Check sheet for the modelled part. Datum: model origin and axes. Units: mm. Face numbers are marked on the shaded views. A direction names the side the tool comes from. Give positions to 0.01 mm unless a question says otherwise; leave off trailing zeros. Order: outer loops, then holes, each group sorted by start corner. A loop starts at its lowest first (then second) coordinate and runs counter-clockwise, first axis right, second up.
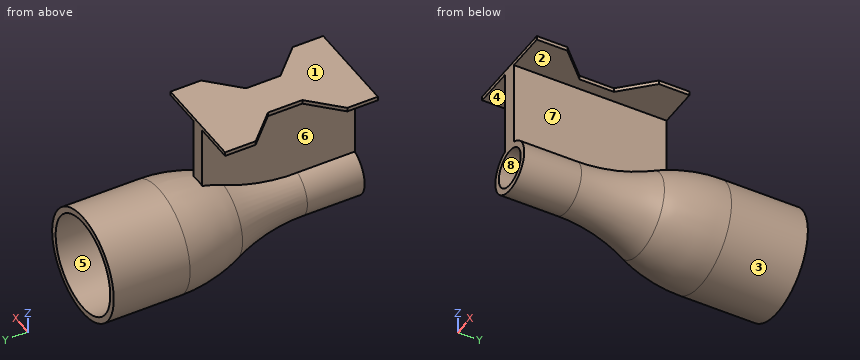
Autodesk Inventor part; units mm, degrees
ref_plane "YZ Plane" through (0, 0, 0) normal (1, 0, 0) x (0, 1, 0)
ref_plane "XZ Plane" through (0, 0, 0) normal (0, 1, 0) x (-1, 0, 0)
ref_plane "XY Plane" through (0, 0, 0) normal (0, 0, 1) x (1, 0, 0)
sketch "Szkic1" plane through (0, 0, 0) normal (1, 0, 0) x (0, 1, 0)
  line L0 (70, 12.5) -> (50, 12.5)
  arc A0 (50, 12.5) -> (35, 9.2857) centre (50, -24.1071) ccw
  arc A1 (15, 5) -> (35, 9.2857) centre (15, 53.8095) ccw
  line L1 (15, 5) -> (0, 5)
  line L2 (0.9785, 0) -> (128.1793, 0) construction
  line L3 (70, 14.1) -> (50, 14.1)
  arc A2 (50, 14.1) -> (34.3444, 10.7452) centre (50, -24.1071) ccw
  arc A3 (15, 6.6) -> (34.3444, 10.7452) centre (15, 53.8095) ccw
  line L4 (15, 6.6) -> (0, 6.6)
  line L5 (70, 14.1) -> (70, 12.5)
  line L6 (0, 6.6) -> (0, 5)
  line L7 (-25.6359, 0) -> (153.8152, 0)
  line L8 (70, 14.1) -> (70, 0)
  line L9 (0, 0) -> (0, 5)
  dimension "d35" = 5
  dimension "d36" = 12.5
  dimension "d37" = 70
  dimension "d38" = 20
  dimension "d39" = 15
  dimension "d40" = 20
  dimension "d41" = 1.6
revolve "Obrót1" add sketch "Szkic1" angle 360 about axis through (0, -10, 0) along (0, 1, 0) contours L0 A0 A1 L1 L6 L4 A3 A2 L3 L5
sketch "Szkic3" plane through (0, 0, 0) normal (0, 1, 0) x (-1, 0, 0)
  line L0 (2.1408, 6.3327) -> (-1.8592, 6.3327)
  line L1 (-1.8592, 6.3327) -> (-1.8592, 28.95)
  line L2 (-1.8592, 28.95) -> (2.1408, 28.95)
  line L3 (2.1408, 28.95) -> (2.1408, 6.3327)
  line L4 (-12.3592, 30) -> (12.6408, 30)
  line L5 (12.6408, 30) -> (12.6408, 28.95)
  line L6 (12.6408, 28.95) -> (-12.3592, 28.95)
  line L7 (-12.3592, 28.95) -> (-12.3592, 30)
  circle A0 centre (0, 0) radius 12.5
  line L8 (2.1408, 12.3153) -> (-1.8592, 12.361)
  circle A1 centre (0, 0) radius 6.6
  point P0 (0.1408, 28.95)
  point P1 (0.1408, 30)
  point P2 (2.1408, 28.95)
  point P3 (-1.8592, 28.95)
  dimension "d17" = 4
  dimension "d19" = 1.05
  dimension "d20" = 25
  dimension "d21" = 30
extrude "Wyciągnięcie proste2" add sketch "Szkic3" along normal blind 40 contours L2 L6 L7 L4 L5
extrude "Wyciągnięcie proste3" add sketch "Szkic3" along normal blind 40 contours L0 A1 L1 L8 L3 | L0 A1 | A0 L1 L2 L3 | L8 A0 picked at (0.2091, 6.4118)
sketch "Szkic4" plane through (0, 40, 0) normal (0, 1, 0) x (1, 0, 0)
  line L0 (-12.6408, -30) -> (12.3592, -30)
  line L1 (1.9943, -30) -> (-2.1408, -30)
  line L2 (-2.1408, -5) -> (1.8592, -5)
  line L3 (-2.1408, -30) -> (1.8592, -30)
  line L4 (1.8592, -30) -> (1.8592, -5)
  line L5 (1.8592, -5) -> (-2.1408, -5)
  line L6 (-2.1408, -5) -> (-2.1408, -30)
  point P0 (0, 0)
  point P1 (-2, -5)
  point P2 (-2, -5)
  point P3 (-0.1408, -30)
  dimension "d42" = 4
  dimension "d43" = 25
extrude "Wyciągnięcie proste4" add sketch "Szkic4" against normal blind 1.2
sketch "Szkic5" plane through (-12.6408, 0, 30) normal (0, 0, 1) x (1, 0, 0)
  line L0 (0, 0) -> (25, 0)
  line L1 (0, 0) -> (0, 8)
  line L2 (0, 0) -> (0, 40)
  line L3 (0, 8) -> (7.5, 15.5)
  line L4 (7.5, 15.5) -> (7.5, 24.5)
  line L5 (9.5, 70) -> (9.5, 0)
  line L6 (7.5, 24.5) -> (0, 32)
  line L7 (0, 40) -> (25, 40)
  line L8 (0, 32) -> (0, 40)
  line L9 (0, 40) -> (25, 40)
  line L10 (25, 0) -> (25, 40)
  line L11 (25, 40) -> (25, 32)
  line L12 (25, 32) -> (17.5, 24.5)
  line L13 (17.5, 24.5) -> (17.5, 15.5)
  line L14 (17.5, 15.5) -> (25, 8)
  line L15 (25, 8) -> (25, 0)
  line L16 (0, 0) -> (25, 0)
  line L17 (12.5, 0) -> (12.5, 40) construction
  line L18 (14.4324, 40) -> (10.5676, 40) construction
  point P0 (12.6408, 0)
  dimension "d29" = 45
  dimension "d30" = 10
  dimension "d31" = 8
  dimension "d32" = 8
extrude "Wyciągnięcie proste5" cut sketch "Szkic5" against normal blind 1.2 contours L2 L6 L4 L3 | L14 L13 L12 L10
revolve "Obrót2" cut sketch "Szkic1" angle 360 about axis through (0, 0.9785, 0) along (0, 1, 0) contours L8 L7 L9 L1 A1 A0 L0
properties part number "rurka_optv2"
(1) Cross-section at B-B on z = 16. Enter the section's corners in (x, y), then the cut area to 3 significant figures.
Response values:
outline: (-2.14, 0) - (1.86, 0) - (1.86, 40) - (-2.14, 40) - close
area: 160 mm2
(2) Set-up check for the marked faces 4, 5, 6, 7 and 8: record each of +Z, -Z, +X, -X, +Y, -Y from which the full face is reachable in a straight line by a thin tool's end or side.
Response values:
face 4: -X, +Y, -Y
face 5: +Y
face 6: -X, -Y
face 7: +X, -Y
face 8: +Y, -Y
(3) Cross-section at A-A on y = 65. Enter the section's corners in (x, z), then the cut area to 3 significant figures.
Response values:
outline: circle Ø28.2 at (0, 0); hole circle Ø25 at (0, 0)
area: 134 mm2
(4) Material ranges on L1, parallel to X at y = 58.25, z = 0; L2, parallel to X at y = 6, z = 0; L3, parallel to Z at x = 2.25, y = 9, recorded low to high.
Response values:
L1: x = -14.1 to -12.5, 12.5 to 14.1
L2: x = -6.6 to -5, 5 to 6.6
L3: z = -6.2 to -4.47, 4.47 to 6.2, 28.95 to 30
(5) Release check for a two-part mould opening along Z. For the marked faces 1, 2 and 3 record: released by +Z, released by -Z, zero draft, split by the parting line, or undercut.
Response values:
face 1: released by +Z
face 2: undercut
face 3: split by the parting line
(6) Gauge pin test, flat ends, axial feed: pin 1 Ø10 at (y, z) = (24, 5) entering from -X; pin 2 Ø1.5 at (y, z) = (48, 11) entering from +X; pin 3 Ø10 at (y, z) = (24.5, 17.5) entering from -X. Record the tip position at first contact, or that the pin passes through.
Response values:
pin 1: stops at x = -8.19
pin 2: stops at x = 9.61
pin 3: stops at x = -2.14
